Autodesk Inventor part; units mm, degrees
ref_plane "YZ Plane" through (0, 0, 0) normal (1, 0, 0) x (0, 1, 0)
ref_plane "XZ Plane" through (0, 0, 0) normal (0, 1, 0) x (-1, 0, 0)
ref_plane "XY Plane" through (0, 0, 0) normal (0, 0, 1) x (1, 0, 0)
sketch "Sketch1" plane through (0, 0, 0) normal (1, 0, 0) x (0, 1, 0)
  line L0 (5, -15.415) -> (5, -19.415)
  line L1 (5, -19.415) -> (-5, -19.415)
  line L2 (5, -20.415) -> (8.7898, -19.1353)
  line L3 (5, -20.415) -> (7.3565, -27.3935)
  line L4 (7.3565, -27.3935) -> (4.6727, -28.2998)
  line L5 (4.6727, -28.2998) -> (2.4715, -21.7812)
  line L6 (2.4715, -21.7812) -> (-5, -21.7812)
  line L7 (-5, -21.7812) -> (-5, -19.415)
  arc A0 (8.7898, -19.1353) -> (5, -15.415) centre (1.7532, -22.5129) ccw
  point P0 (0, 0)
  point P1 (0, -20.415)
  dimension "d0" = 4
  dimension "d4" = 4
extrude "Extrusion1" add sketch "Sketch1" along normal blind 330
properties part number "junta controler"
Model file for the job. Use its own axes, mm. A direction names the side the tool comes from. Give positions to 0.01 mm unless a question says otherwise; leave off trailing zeros. Order: outer loops, then holes, each group sorted by start corner. A loop starts at its lowest first (then second) coordinate and runs counter-clockwise, first axis right, second up. Notation, with made-up numbers: M 5,80.25 L 32,80.25 A22 ccw 32,116.25 Z; hole C 54.25,-36 d4. An arc over 180 degrees is marked long. Put each result on its own line as item: value. Start each with the question number.
(1) Drill centre lines: L1, parallel to Z at x = 36, y = 1.5 (3 decimals); L2, parallel to Z at x = 149, y = 4.75 (3 decimals); L3, parallel to Y at x = 190.5, z = -23. Where is each one in solid material? Low to high. Write a range as [from, to].
(2) Pin check, flat tips, straight feed: pin 1 Ø5 at (x, z) = (130.5, -25.5) entering from +Y; pin 2 Ø1.2 at (x, z) = (236.5, -17) entering from -Y; pin 3 Ø1 at (x, z) = (124, -22) entering from +Y; pin 4 Ø3 at (y, z) = (2.5, -19) entering from +X. Stop position of each tip, or through.
(3) Band-saw the part on C-C on z = -24.25. Give the cut face in (x, y) (3 decimals).
(4) Tool access for faces 1 (the face through (162.69, 6.162, -23.855)), 2 (the face through (163, 0, -19.415)), 3 (the face through (163, -1, -21.781)): list every direction of +Z, -Z, +X, -X, +Y, -Y with a clear straight run to the whole face (end or side of a thin tool).
(5) Band-saw the part on B-B on y = -1.5. Give the cut face in (x, z) (3 decimals), then the cut area to 3 significant figures.
(6) Band-saw the part on A-A on x = 146. Give the cut face in (y, z) (1 decimal).
Results below:
1. L1: z = [-21.781, -19.415]
1. L2: z = [-28.274, -19.415]
1. L3: y = [2.88, 5.87]
2. pin 1: stops at y = 7.36
2. pin 2: stops at y = 5
2. pin 3: stops at y = 5.7
2. pin 4: stops at x = 330
3. outline: M 0,3.305 L 330,3.305 L 330,6.295 L 0,6.295 Z
4. face 1: +X, -X, +Y
4. face 2: +Z, +X, -X, -Y
4. face 3: -Z, +X, -X, -Y
5. outline: M 0,-21.781 L 330,-21.781 L 330,-19.415 L 0,-19.415 Z
5. area: 781 mm2
6. outline: M -5,-21.8 L 2.5,-21.8 L 4.7,-28.3 L 7.4,-27.4 L 5,-20.4 L 8.8,-19.1 A7.8 ccw 5,-15.4 L 5,-19.4 L -5,-19.4 Z
